Answer from the drawing. Dimensions are ordinates in mm from the lowest x, y and z of the part. A direction names the side the tool comes from. Give positions to 0.01 mm unless a question says otherwise; leave off trailing zeros. Write each loop counter-clockwise with the first axis right and the second up, starting at its lowest first coordinate (ties: lowest second). Pieces come first, ordered by that corner, then holes.
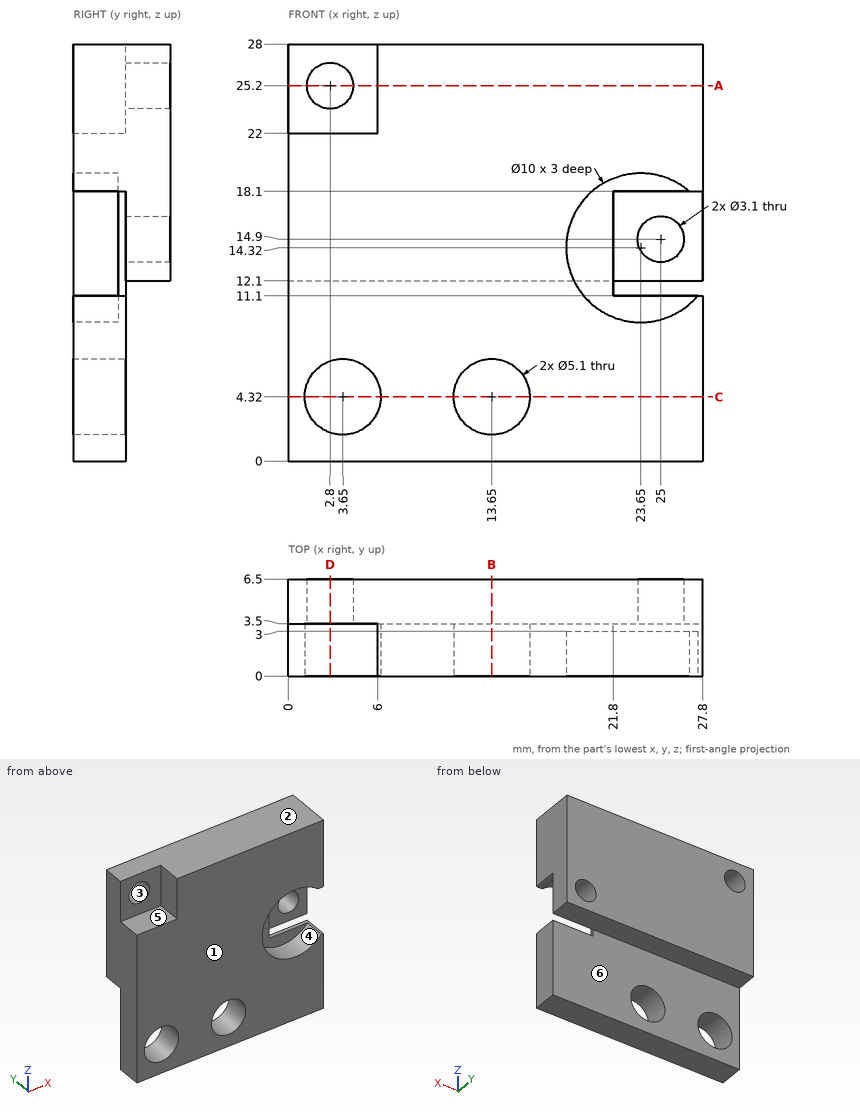
Item 1: Section A-A (z = 25.2) is taken. Write down the section's boundary in (x, y), and give its area (3 significant figures).
Result set:
outline: (0, 3.5) - (1.25, 3.5) - (1.25, 6.5) - (0, 6.5) - close; (4.35, 3.5) - (6, 3.5) - (6, 0) - (27.8, 0) - (27.8, 6.5) - (4.35, 6.5) - close
area: 150 mm2
Item 2: Each of these flat-tipped pins is pushed along its axis until it touches: pin 1 Ø2 at (y, z) = (5.5, 6.5) entering from -X; pin 2 Ø1 at (y, z) = (1.5, 26) entering from -X; pin 3 Ø3.5 at (x, z) = (2.8, 25.2) entering from -Y; pin 4 Ø6 at (x, z) = (3.65, 4.32) entering from +Y. Where does it stop, or does it pass through?
Result set:
pin 1: passes through
pin 2: stops at x = 6
pin 3: stops at y = 3.5
pin 4: stops at y = 3.5
Item 3: Section C-C (z = 4.32) is taken. Write down the section's boundary in (x, y).
Result set:
outline: (0, 0) - (1.1, 0) - (1.1, 3.5) - (0, 3.5) - close; (6.2, 0) - (11.1, 0) - (11.1, 3.5) - (6.2, 3.5) - close; (16.2, 0) - (27.8, 0) - (27.8, 3.5) - (16.2, 3.5) - close
Item 4: Find the intervals of material crossed by line 1 along X through (y, z) = (1.05, 4.32); line 2 along Z through (x, y) = (23.65, 2.2); line 3 along Y through (x, z) = (10.5, 11.75), in increasing order.
Result set:
line 1: x = 0 to 1.1, 6.2 to 11.1, 16.2 to 27.8
line 2: z = 0 to 9.32, 19.32 to 28
line 3: y = 0 to 3.5
Item 5: Determine the mould class of the marked faces 1, 2 and 3 for opening direction Z: pulls with the +Z half, pulls with the -Z half, needs draft (parallel to the pull), parting line crosses it, or undercut.
Result set:
face 1: needs draft
face 2: pulls with the +Z half
face 3: undercut
Item 6: Which of the six approach directions +Z, -Z, +X, -X, +Y, -Y give full straight-line access (tool end or side, diameter ignored) to the marked faces 4, 5 and 6?
Result set:
face 4: -Y
face 5: +Z, -X, -Y
face 6: -Z, +X, -X, +Y
Item 7: Section D-D (x = 2.8) is taken. Write down the section's boundary in (y, z).
Result set:
outline: (0, 0) - (3.5, 0) - (3.5, 1.92) - (0, 1.92) - close; (0, 6.72) - (3.5, 6.72) - (3.5, 12.1) - (6.5, 12.1) - (6.5, 23.65) - (3.5, 23.65) - (3.5, 22) - (0, 22) - close; (3.5, 26.75) - (6.5, 26.75) - (6.5, 28) - (3.5, 28) - close
Item 8: Section B-B (x = 13.65) is taken. Write down the section's boundary in (y, z), and give its area (3 significant figures).
Result set:
outline: (0, 0) - (3.5, 0) - (3.5, 1.77) - (0, 1.77) - close; (0, 6.87) - (3.5, 6.87) - (3.5, 12.1) - (6.5, 12.1) - (6.5, 28) - (0, 28) - close
area: 128 mm2
